Input: dimensioned drawing with shaded views. Units: mm. Origin: part minimum x, y, z. Give positions to 0.01 mm unless a question says otherwise; leave off trailing zeros. Order: outer loops, then holes, each group sorted by start corner. A loop starts at its lowest first (then second) coordinate and runs counter-clockwise, first axis right, second up. Notation, with made-up numbers: (47.5, 16.5) - (97.5, 16.5) arc R28 ccw to (97.5, 53.5) - close; hole circle Ø8 at (50.25, -8). An arc over 180 degrees is marked (long way). Use a Markdown table: item, result.
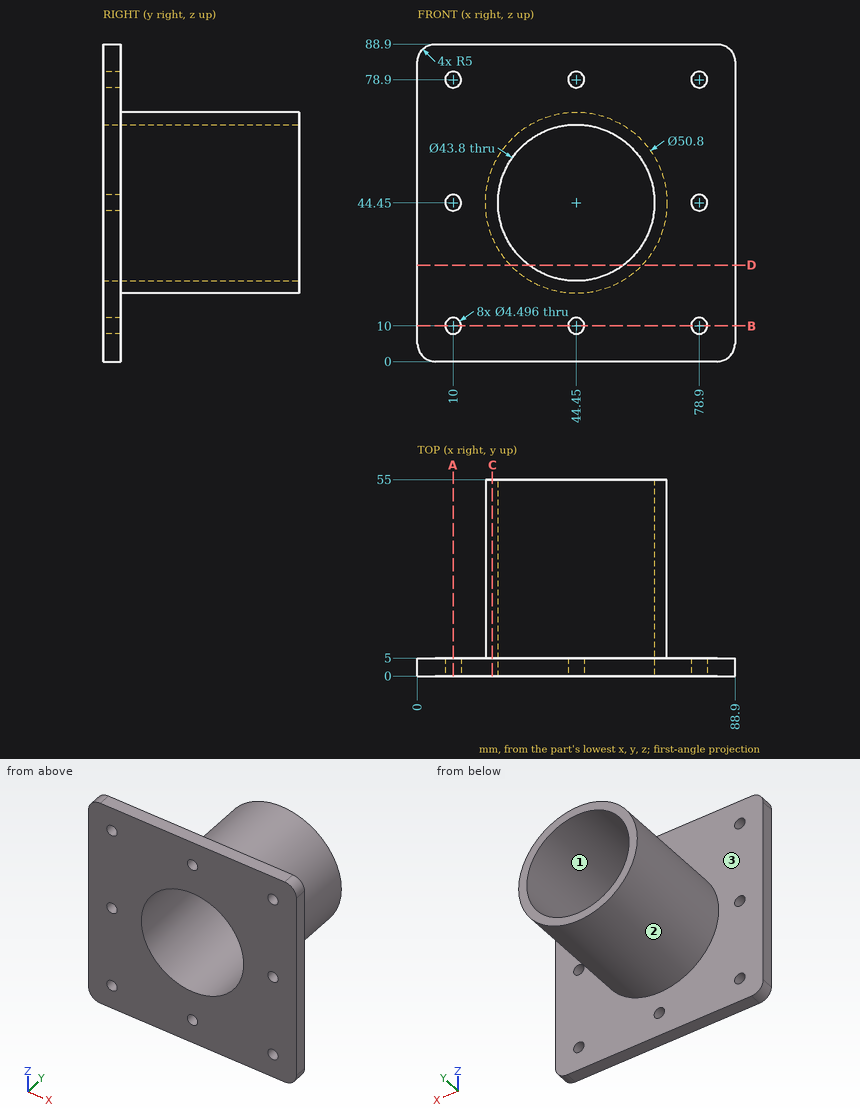
1. Pin query (flat end, axial travel): pin 1 (6 mm diameter, centred on x = 10, z = 10, fed in from +Y); pin 2 (4 mm diameter, centred on y = 41.5, z = 42.5, fed in from +X); pin 3 (10 mm diameter, centred on x = 11.5, z = 30.5, fed in from -Y); pin 4 (3.5 mm diameter, centred on x = 10, z = 78.9, fed in from +Y). Return the tip coordinate at first contact, or that it passes through.
Response:
| item | result |
|---|---|
| pin 1 | stops at y = 5 |
| pin 2 | stops at x = 69.85 |
| pin 3 | stops at y = 0 |
| pin 4 | passes through |
2. Section query C-C (x = 21). Return loops of the section in (y, z), then the cut area to 3 significant figures.
Response:
| item | result |
|---|---|
| outline | (0, 0) - (5, 0) - (5, 34.69) - (55, 34.69) - (55, 54.21) - (5, 54.21) - (5, 88.9) - (0, 88.9) - close |
| area | 1,420 mm^2 |
3. Material intervals for line 1 along Z through (x, y) = (78.9, 2.1); line 2 along X through (y, z) = (3, 44), sorted ascending.
Response:
| item | result |
|---|---|
| line 1 | z = 0 to 7.75, 12.25 to 42.2, 46.7 to 76.65, 81.15 to 88.9 |
| line 2 | x = 0 to 7.8, 12.2 to 22.55, 66.35 to 76.7, 81.1 to 88.9 |
4. Mould query, pull axis Z, two halves, no side actions, for the marked faces 1, 2 and 3. Classes: pulls with the +Z half, pulls with the -Z half, needs draft (parallel to the pull), parting line crosses it, or undercut.
Response:
| item | result |
|---|---|
| face 1 | undercut |
| face 2 | parting line crosses it |
| face 3 | needs draft |
5. Section query B-B (z = 10). Return loops of the section in (x, y).
Response:
| item | result |
|---|---|
| outline | (0, 0) - (7.75, 0) - (7.75, 5) - (0, 5) - close; (12.25, 0) - (42.2, 0) - (42.2, 5) - (12.25, 5) - close; (46.7, 0) - (76.65, 0) - (76.65, 5) - (46.7, 5) - close; (81.15, 0) - (88.9, 0) - (88.9, 5) - (81.15, 5) - close |
6. Section query A-A (x = 10). Return loops of the section in (y, z).
Response:
| item | result |
|---|---|
| outline | (0, 0) - (5, 0) - (5, 7.75) - (0, 7.75) - close; (0, 12.25) - (5, 12.25) - (5, 42.2) - (0, 42.2) - close; (0, 46.7) - (5, 46.7) - (5, 76.65) - (0, 76.65) - close; (0, 81.15) - (5, 81.15) - (5, 88.9) - (0, 88.9) - close |
7. Section query D-D (z = 27). Return loops of the section in (x, y), then the cut area to 3 significant figures.
Response:
| item | result |
|---|---|
| outline | (0, 0) - (31.22, 0) - (31.22, 55) - (25.99, 55) - (25.99, 5) - (0, 5) - close; (57.68, 0) - (88.9, 0) - (88.9, 5) - (62.91, 5) - (62.91, 55) - (57.68, 55) - close |
| area | 835 mm^2 |
